Study the drawing (mm; zero at the part's minimum x, y, z) and answer. A direction names the side the tool comes from. Coordinates: 2 decimals unless noted, no trailing zeros. Order: outer loops, then holes, each group sorted by start corner. A loop starts at its lowest first (then second) coordinate and runs counter-clockwise, first axis right, second up.
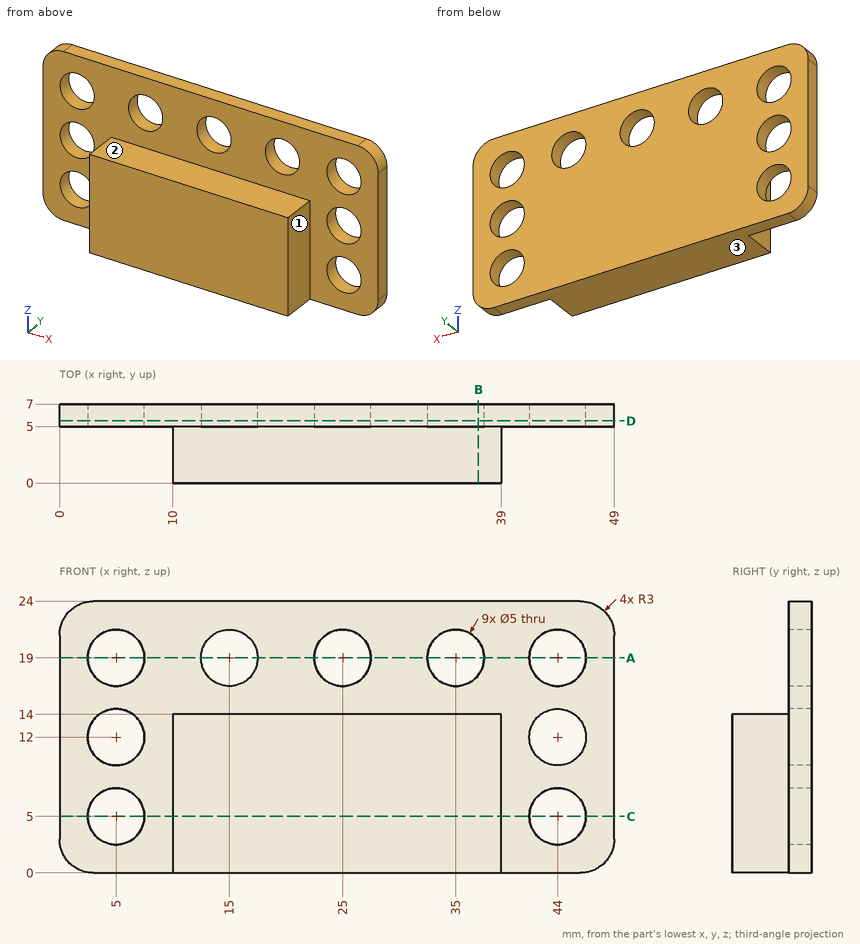
(1) Find section D-D (y = 5.5). Give the number of separate pieces and of enclosed holes in the cut face, and give its area (3 significant figures).
(2) Each of these flat-tipped pins is pushed along its axis until it touches: pin 1 Ø2.5 at (x, y) = (28.5, 1.5) entering from +Z; pin 2 Ø6 at (x, z) = (15, 19) entering from -Y; pin 3 Ø1.5 at (y, z) = (3.5, 7.5) entering from +X; pin 4 Ø4.5 at (x, z) = (5, 5) entering from +Y. Where does it stop, or does it pass through?
(3) For the marked faces 1, 2 and 3, determine the directions among +Z, -Z, +X, -X, +Y, -Y from which every point of the face is accessible in a straight line to the end or side of a thin tool.
(4) Find section A-A (z = 19). Write down the section's boundary in (x, y), and give its area (3 significant figures).
(5) Find section C-C (z = 5). Write down the section's boundary in (x, y), and give its area (3 significant figures).
(6) Find section B-B (x = 37). Write down the section's boundary in (y, z), and give its area (3 significant figures).
(7) Consider line 1 (X direction, y = 5.75, z = 19); line 2 (Z direction, x = 44, y = 5.75); line 3 (X direction, y = 6.35, z = 5). Determine where each line is inside the solid, lowest interval first.
Findings below:
1. separate pieces: 1
1. enclosed holes: 9
1. area: 992 mm2
2. pin 1: stops at z = 14
2. pin 2: stops at y = 5
2. pin 3: stops at x = 39
2. pin 4: passes through
3. face 1: +Z, -Z, +X, -Y
3. face 2: +Z, +X, -X, -Y
3. face 3: -Z, +X, -X, +Y, -Y
4. outline: (0, 5) - (2.5, 5) - (2.5, 7) - (0, 7) - close; (7.5, 5) - (12.5, 5) - (12.5, 7) - (7.5, 7) - close; (17.5, 5) - (22.5, 5) - (22.5, 7) - (17.5, 7) - close; (27.5, 5) - (32.5, 5) - (32.5, 7) - (27.5, 7) - close; (37.5, 5) - (41.5, 5) - (41.5, 7) - (37.5, 7) - close; (46.5, 5) - (49, 5) - (49, 7) - (46.5, 7) - close
4. area: 48.0 mm2
5. outline: (0, 5) - (2.5, 5) - (2.5, 7) - (0, 7) - close; (7.5, 5) - (10, 5) - (10, 0) - (39, 0) - (39, 5) - (41.5, 5) - (41.5, 7) - (7.5, 7) - close; (46.5, 5) - (49, 5) - (49, 7) - (46.5, 7) - close
5. area: 223 mm2
6. outline: (0, 0) - (7, 0) - (7, 17.5) - (5, 17.5) - (5, 14) - (0, 14) - close; (5, 20.5) - (7, 20.5) - (7, 24) - (5, 24) - close
6. area: 112 mm2
7. line 1: x = 0 to 2.5, 7.5 to 12.5, 17.5 to 22.5, 27.5 to 32.5, 37.5 to 41.5, 46.5 to 49
7. line 2: z = 0 to 2.5, 7.5 to 9.5, 14.5 to 16.5, 21.5 to 24
7. line 3: x = 0 to 2.5, 7.5 to 41.5, 46.5 to 49
